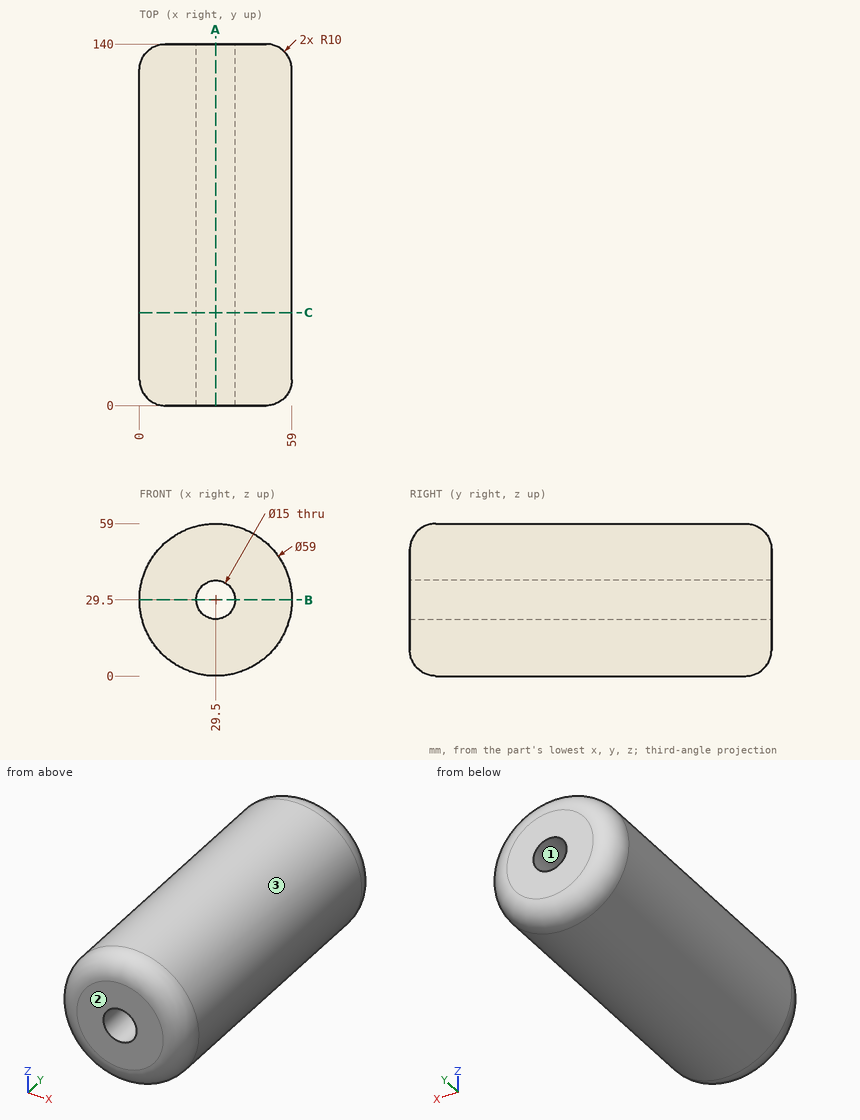
Input: dimensioned drawing with shaded views. Units: mm. Origin: part minimum x, y, z. Round coordinates to 2 decimals unless told otherwise and drop trailing zeros. Loops run counter-clockwise (first coordinate to the right, second up) from the corner with the lowest first, then second, coordinate; pieces in that order, holes last. Notation, with made-up numbers: M 63.5,-18.75 L 102.5,-18.75 A25 ccw 102.5,3.25 Z; hole C 59.5,-6.75 d8. An arc over 180 degrees is marked long. Answer in a Markdown table with one row per item. Add a question column.
1. Section B-B (z = 29.5). Output: boundary loops of the cut face in (x, y).
2. Contact query for flat-ended pins moving along their axis: pin 1 (4 mm diameter, centred on x = 48.5, y = 70.5, fed in from -Z); pin 2 (1.5 mm diameter, centred on x = 31, y = 78, fed in from -Z); pin 3 (1 mm diameter, centred on x = 52, z = 34, fed in from +Y). Output: stop coordinate, or through.
3. Section C-C (y = 36). Output: boundary loops of the cut face in (x, z).
4. Ray query, probe 1 along X at (y, z) = (42.5, 30); probe 2 along X at (y, z) = (16, 23.5). Return the intervals inside material, ascending.
5. Mould query, pull axis X, two halves, no side actions, for the marked faces 1, 2 and 3. Classes: released by +X, released by -X, zero draft, split by the parting line, or undercut.
6. Section A-A (x = 29.5). Output: boundary loops of the cut face in (y, z), and give its area (3 significant figures).
Values follow:
| question | item | result |
|---|---|---|
| 1 | outline | M 0,10 A10 ccw 10,0 L 22,0 L 22,140 L 10,140 A10 ccw 0,130 Z; M 37,0 L 49,0 A10 ccw 59,10 L 59,130 A10 ccw 49,140 L 37,140 Z |
| 2 | pin 1 | z = 5.39 |
| 2 | pin 2 | z = 0.01 |
| 2 | pin 3 | y = 139.56 |
| 3 | outline | C 29.5,29.5 d59; hole C 29.5,29.5 d15 |
| 4 | probe 1 | 0 to 22.02, 36.98 to 59 |
| 4 | probe 2 | 0.62 to 25, 34 to 58.38 |
| 5 | face 1 | undercut |
| 5 | face 2 | zero draft |
| 5 | face 3 | split by the parting line |
| 6 | outline | M 0,10 A10 ccw 10,0 L 130,0 A10 ccw 140,10 L 140,22 L 0,22 Z; M 0,37 L 140,37 L 140,49 A10 ccw 130,59 L 10,59 A10 ccw 0,49 Z |
| 6 | area | 6,070 mm^2 |
